Can you work these out from the drawing? Everything is in mm from the part's minimum corner. Round coordinates to 2 decimals unless told otherwise and drop trailing zeros. Write each loop counter-clockwise with the first axis right and the second up, starting at its lowest first coordinate (ties: lowest second). Pieces come first, ordered by that corner, then holes. Notation, with made-up numbers: (68.5, 59.5) -> (86.5, 59.5) arc R4 cw to (86.5, 66.5) -> close; hole circle Ø7 at (79, 49.5). An arc over 180 degrees is marked (long way). Answer as CSV lines item,"result". Start each with the question number.
Q1. Will these pins go through, and if not, where does the flat tip stop? pin 1 Ø1.4 at (y, z) = (1, 1) entering from +X; pin 2 Ø0.8 at (x, y) = (126.5, 0.5) entering from -Z; pin 3 Ø1 at (x, y) = (75.5, 1) entering from +Z.
Q2. If I drill on line 1 (X direction, y = 0.45, z = 38); line 2 (X direction, y = 1.25, z = 27.5); line 3 (Z direction, x = 44.5, y = 1.7), over which ranges is the centre line in solid material (lowest first)? Write a range as [from, to].
Q3. Imagine slicing it at A-A on z = 26. Please give me the cut outline in (x, y), and give its area (3 significant figures).
Q4. Imagine slicing it at B-B on x = 19.5. Please give me the cut outline in (y, z).
Q5. Imagine slicing it at C-C on z = 35. Please give me the cut outline in (x, y).
Q6. Imagine slicing it at D-D on y = 1.9. Please give me the cut outline in (x, z).
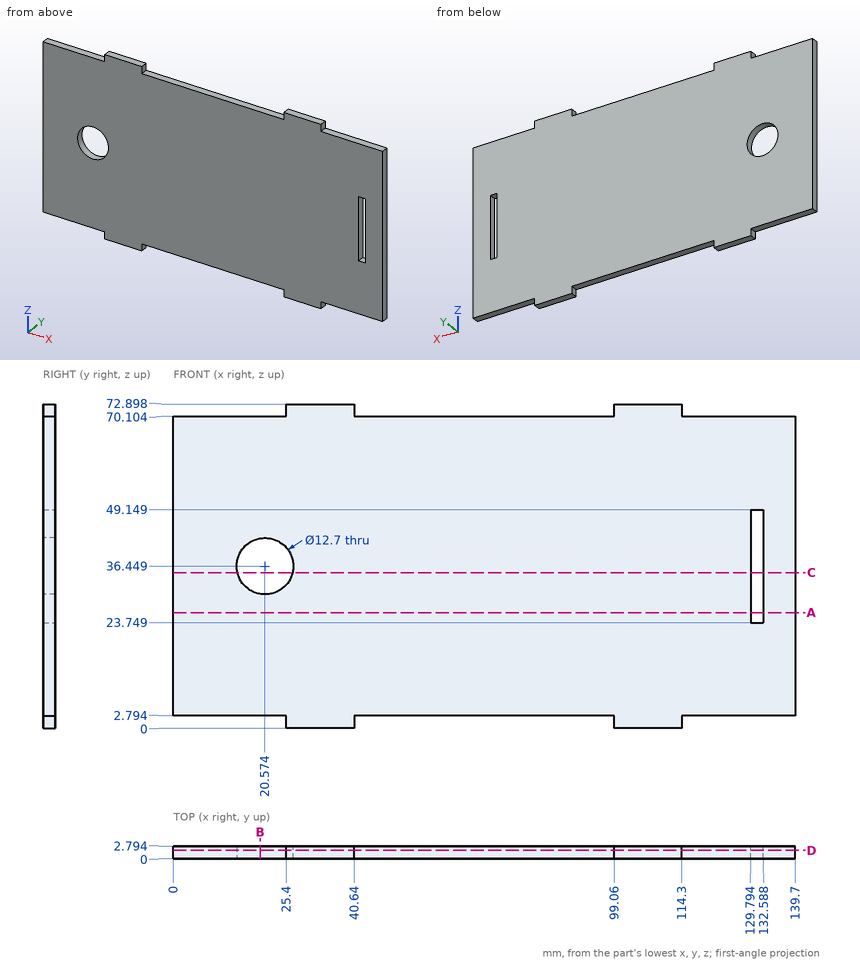
Checks:
1,pin 1,"x = 114.3"
1,pin 2,"z = 2.79"
1,pin 3,"z = 70.1"
2,line 1,"[0, 14.42], [26.73, 129.79], [132.59, 139.7]"
2,line 2,"[0, 129.79], [132.59, 139.7]"
2,line 3,"[2.79, 70.1]"
3,outline,"(0, 0) -> (129.79, 0) -> (129.79, 2.79) -> (0, 2.79) -> close; (132.59, 0) -> (139.7, 0) -> (139.7, 2.79) -> (132.59, 2.79) -> close"
3,area,"383 mm^2"
4,outline,"(0, 2.79) -> (2.79, 2.79) -> (2.79, 30.19) -> (0, 30.19) -> close; (0, 42.71) -> (2.79, 42.71) -> (2.79, 70.1) -> (0, 70.1) -> close"
5,outline,"(0, 0) -> (14.39, 0) -> (14.39, 2.79) -> (0, 2.79) -> close; (26.76, 0) -> (129.79, 0) -> (129.79, 2.79) -> (26.76, 2.79) -> close; (132.59, 0) -> (139.7, 0) -> (139.7, 2.79) -> (132.59, 2.79) -> close"
6,outline,"(0, 2.79) -> (25.4, 2.79) -> (25.4, 0) -> (40.64, 0) -> (40.64, 2.79) -> (99.06, 2.79) -> (99.06, 0) -> (114.3, 0) -> (114.3, 2.79) -> (139.7, 2.79) -> (139.7, 70.1) -> (114.3, 70.1) -> (114.3, 72.9) -> (99.06, 72.9) -> (99.06, 70.1) -> (40.64, 70.1) -> (40.64, 72.9) -> (25.4, 72.9) -> (25.4, 70.1) -> (0, 70.1) -> close; hole circle Ø12.7 at (20.57, 36.45); hole (129.79, 23.75) -> (132.59, 23.75) -> (132.59, 49.15) -> (129.79, 49.15) -> close"
